```python
from build123d import *

# Parameters (mm, degrees)
EXTRUDE_1_DEPTH     = 20
SKETCH_2_W          = 17
SKETCH_2_H          = 10
CUT_EXTRUDE_1_DEPTH = 11
CUT_EXTRUDE_2_REACH = 18
CHAMFER_1_SIZE      = 3
CHAMFER_2_SIZE      = 2
CHAMFER_2_SIZE2     = 2.383507185
CUT_EXTRUDE_3_DEPTH = 2
CUT_EXTRUDE_4_DEPTH = 2
SKETCH_5_R          = 0.5
CUT_EXTRUDE_5_DEPTH = 6


with BuildPart() as part:
    # Эскиз1 → Бобышка-Вытянуть1 (new body)
    with BuildSketch(Plane.XY):
        Polygon((0, 0), (1, 0), (1, -9), (4, -9), (4, 11), (-12, 11), (-12, 1), (0, 1), align=None)
    extrude(amount=EXTRUDE_1_DEPTH)

    # Эскиз2 → Вырез-Вытянуть1 (cut)
    with BuildSketch(Plane.ZY.offset(12)):
        with Locations((11.5, 6)):
            Rectangle(SKETCH_2_W, SKETCH_2_H)
    extrude(amount=-CUT_EXTRUDE_1_DEPTH, mode=Mode.SUBTRACT)

    # Эскиз3 → Вырез-Вытянуть2 (cut, up to next)
    with BuildSketch(Plane(origin=(4, 0, 0), x_dir=(0, 0, -1), z_dir=(1, 0, 0)), mode=Mode.PRIVATE) as cut_extrude_2_sk1:
        with BuildLine():
            Line((-12.75, -2.4), (-11.25, -2.4))
            ThreePointArc((-11.25, -2.4), (-9.65, -4), (-11.25, -5.6))
            Line((-11.25, -5.6), (-12.75, -5.6))
            ThreePointArc((-12.75, -5.6), (-14.35, -4), (-12.75, -2.4))
        make_face()
    cut_extrude_2_tool1 = extrude(cut_extrude_2_sk1.sketch, amount=-CUT_EXTRUDE_2_REACH, mode=Mode.PRIVATE) & part.part
    add(cut_extrude_2_tool1.solids().sort_by_distance((4, -4, 12))[0], mode=Mode.SUBTRACT)

    # Фаска1
    chamfer_1_edges = [part.edges().sort_by_distance(p)[0] for p in [
        (4, 11, 10),
    ]]
    chamfer(chamfer_1_edges, length=CHAMFER_1_SIZE)

    # Фаска2
    chamfer_2_edges = [part.edges().sort_by_distance(p)[0] for p in [
        (-12, 11, 1.5),
    ]]
    chamfer_2_side = [part.faces().sort_by_distance(p)[0] for p in [
        (-12, 6, 1.5),
    ]]
    chamfer(chamfer_2_edges, length=CHAMFER_2_SIZE, length2=CHAMFER_2_SIZE2, reference=chamfer_2_side[0])

    # Эскиз3<3> → Вырез-Вытянуть3 (cut)
    with BuildSketch(Plane(origin=(4, 0, 0), x_dir=(0, 0, -1), z_dir=(1, 0, 0))):
        with BuildLine():
            Line((-12.75, -0.75), (-11.25, -0.75))
            ThreePointArc((-11.25, -0.75), (-8, -4), (-11.25, -7.25))
            Line((-11.25, -7.25), (-12.75, -7.25))
            ThreePointArc((-12.75, -7.25), (-16, -4), (-12.75, -0.75))
        make_face()
        with BuildLine():
            Line((-12.75, -2.4), (-11.25, -2.4))
            ThreePointArc((-11.25, -2.4), (-9.65, -4), (-11.25, -5.6))
            Line((-11.25, -5.6), (-12.75, -5.6))
            ThreePointArc((-12.75, -5.6), (-14.35, -4), (-12.75, -2.4))
        make_face(mode=Mode.SUBTRACT)
    extrude(amount=-CUT_EXTRUDE_3_DEPTH, mode=Mode.SUBTRACT)

    # Эскиз4 → Вырез-Вытянуть4 (cut)
    with BuildSketch(Plane(origin=(4, 0, 0), x_dir=(0, 0, -1), z_dir=(1, 0, 0))):
        with BuildLine():
            Line((-20, 1), (-6, 1))
            ThreePointArc((-6, 1), (-3.171572875, 2.171572875), (-2, 5))
            Line((-2, 5), (-2, 11))
            Line((-2, 11), (-20, 11))
            Line((-20, 11), (-20, 10))
            Line((-20, 10), (-20, 1))
        make_face()
    extrude(amount=-CUT_EXTRUDE_4_DEPTH, mode=Mode.SUBTRACT)

    # Эскиз5 → Вырез-Вытянуть5 (cut, through all)
    with BuildSketch(Plane.ZY.offset(1)):
        with Locations((4, 8.5)):
            Circle(SKETCH_5_R)
        with Locations((5.5, 6.75)):
            Circle(SKETCH_5_R)
        with Locations((5.5, 5.25)):
            Circle(SKETCH_5_R)
        with Locations((4, 3.5)):
            Circle(SKETCH_5_R)
    extrude(amount=-CUT_EXTRUDE_5_DEPTH, mode=Mode.SUBTRACT)


solid = part.part
```
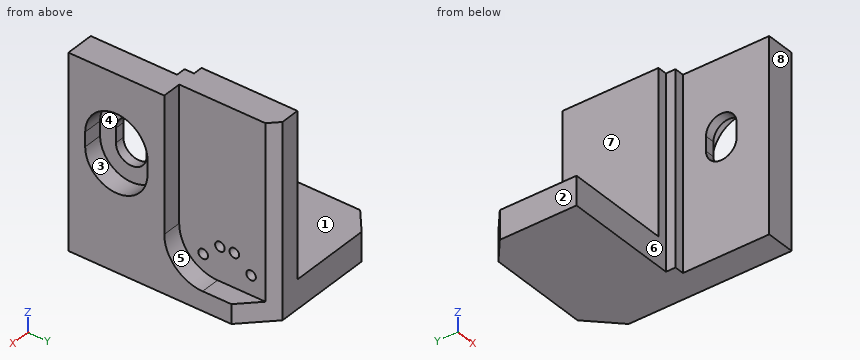
Input: part model. Units: mm. Frame: model coordinates. Face numbers are marked on the shaded views. A direction names the side the tool comes from. Round coordinates to 2 decimals unless told otherwise and drop trailing zeros. Loops run counter-clockwise (first coordinate to the right, second up) from the corner with the lowest first, then second, coordinate; pieces in that order, holes last. Notation, with made-up numbers: (56, -22) -> (97, -22) arc R20 cw to (97, -9) -> close; hole circle Ø11 at (5, 73.25). An arc over 180 degrees is marked (long way). Use one line per item in the form item = value. Start each with the question number.
Item 1: Section query B-B on x = -0.5. Return the cut outline in (y, z), then the cut area to 3 significant figures.
Item 2: Mould query, pull axis Z, two halves, no side actions, for the marked faces 1, 2 and 3. Classes: pulls with the +Z half, pulls with the -Z half, needs draft (parallel to the pull), parting line crosses it, or undercut.
Item 3: Section query D-D on y = -4. Return the cut outline in (x, z).
Item 4: Section query A-A on y = 8.5. Return the cut outline in (x, z), then the cut area to 3 significant figures.
Item 5: Set-up query: the marked faces 4, 5, 6, 7 and 8. Return all of +Z, -Z, +X, -X, +Y, -Y with unobstructed straight access to the full face (end or side cutting, diameter ignored); none if empty.
Item 6: Contact query for flat-ended pins moving along their axis: pin 1 Ø3 at (y, z) = (8.5, 15.5) entering from -X; pin 2 Ø5 at (x, y) = (-8, 6.5) entering from +Z; pin 3 Ø6 at (x, y) = (-4, -6) entering from +Z; pin 4 Ø1.6 at (x, y) = (3, 8) entering from +Z. Output: stop coordinate, or through.
Item 7: Section query C-C on z = 5.5. Return the cut outline in (x, y), then the cut area to 3 significant figures.
Item 8: Material intervals for L1, parallel to Y at x = 0.75, z = 5.5; L2, parallel to Y at x = 3, z = 12.75; L3, parallel to Y at x = -0.5, z = 1.5, sorted ascending. Write a range as from..to.
Ans:
q1.outline = (1, 0) -> (11, 0) -> (11, 20) -> (1, 20) -> close; hole circle Ø1 at (3.5, 4); hole circle Ø1 at (5.25, 5.5); hole circle Ø1 at (6.75, 5.5); hole circle Ø1 at (8.5, 4)
q1.area = 197 mm^2
q2.face_1 = pulls with the +Z half
q2.face_2 = needs draft
q2.face_3 = undercut
q3.outline = (1, 0) -> (4, 0) -> (4, 8) -> (2, 8) -> (2, 9.65) -> (1, 9.65) -> close; (1, 14.35) -> (2, 14.35) -> (2, 16) -> (4, 16) -> (4, 20) -> (1, 20) -> close
q4.outline = (-12, 0) -> (3.5, 0) -> (3.5, 2) -> (2, 2) -> (2, 3.5) -> (-1, 3.5) -> (-1, 3) -> (-12, 3) -> close; (-1, 4.5) -> (2, 4.5) -> (2, 20) -> (-1, 20) -> close
q4.area = 93.0 mm^2
q5.face_4 = +X
q5.face_5 = +Z, +X, +Y
q5.face_6 = +Z, -Z, -X, -Y
q5.face_7 = +Z, -X, +Y, -Y
q5.face_8 = +Z, -Z, +X, -X, -Y
q6.pin_1 = -1
q6.pin_2 = 3
q6.pin_3 = through
q6.pin_4 = 2
q7.outline = (-1, 1) -> (0, 1) -> (0, 0) -> (1, 0) -> (1, -9) -> (4, -9) -> (4, 1.03) -> (2, 1.03) -> (2, 4.75) -> (-1, 4.75) -> close; (-1, 5.75) -> (2, 5.75) -> (2, 6.25) -> (-1, 6.25) -> close; (-1, 7.25) -> (2, 7.25) -> (2, 10) -> (1, 11) -> (-1, 11) -> close
q7.area = 54.6 mm^2
q8.L1 = 0..4.75, 5.75..6.25, 7.25..11
q8.L2 = -9..-7.25, -0.75..1
q8.L3 = 1..11
